Work out the finished part from the listing and answer in its coordinate system (mm). Coordinates: 2 decimals unless noted, no trailing zeros. Order: outer loops, then holes, each group sorted by start corner. A loop starts at its lowest first (then second) coordinate and runs counter-clockwise, first axis right, second up.
```python
from build123d import *

# Parameters (mm, degrees)
CROQUIS1_R              = 6.35
SALIENTE_EXTRUIR1_DEPTH = 12
CROQUIS2_R              = 52.802243625
CROQUIS2_R_2            = 9.5
CORTAR_EXTRUIR1_DEPTH   = 12
CORTAR_EXTRUIR1_DRAFT   = -55
CROQUIS3_R              = 41.337917096
CROQUIS3_R_2            = 9.5
CORTAR_EXTRUIR2_DEPTH   = 12
CORTAR_EXTRUIR2_DRAFT   = -63
CORTAR_EXTRUIR3_REACH   = 20.83
MATRIZC1_COUNT          = 6


with BuildPart() as part:
    # Croquis1 → Saliente-Extruir1 (new body)
    with BuildSketch(Plane(origin=(0, 0, 0), x_dir=(1, 0, 0), z_dir=(0, 1, 0))):
        Polygon((10.969655115, 0), (5.484827557, 9.5), (-5.484827557, 9.5), (-10.969655115, 0), (-5.484827557, -9.5), (5.484827557, -9.5), align=None)
        with Locations(Location((0, 0, 0), (0, 0, 270))):
            Circle(CROQUIS1_R, mode=Mode.SUBTRACT)
    extrude(amount=SALIENTE_EXTRUIR1_DEPTH)


with BuildPart() as cortar_extruir1_tool:
    # Croquis2 → Cortar-Extruir1 (with draft: the straight prism first)
    with BuildSketch(Plane(origin=(0, 12, 0), x_dir=(1, 0, 0), z_dir=(0, 1, 0))):
        Circle(CROQUIS2_R)
        Circle(CROQUIS2_R_2, mode=Mode.SUBTRACT)
    extrude(amount=-CORTAR_EXTRUIR1_DEPTH)
    # Cortar-Extruir1: the draft: its side faces are tilted about the plane it starts from
    cortar_extruir1_sides = [cortar_extruir1_tool.faces().sort_by_distance(p)[0] for p in [
        (-52.802243625, 6, 0),
        (-9.5, 6, 0),
    ]]
    draft(cortar_extruir1_sides, Plane(origin=(0, 12, 0), x_dir=(1, 0, 0), z_dir=(0, 1, 0)), CORTAR_EXTRUIR1_DRAFT)


with BuildPart() as part_1:
    add(part.part)

    # Cortar-Extruir1: cut by cortar_extruir1_tool
    add(cortar_extruir1_tool.part, mode=Mode.SUBTRACT)


with BuildPart() as cortar_extruir2_tool:
    # Croquis3 → Cortar-Extruir2 (with draft: the straight prism first)
    with BuildSketch(Plane.XZ):
        Circle(CROQUIS3_R)
        Circle(CROQUIS3_R_2, mode=Mode.SUBTRACT)
    extrude(amount=-CORTAR_EXTRUIR2_DEPTH)
    # Cortar-Extruir2: the draft: its side faces are tilted about the plane it starts from
    cortar_extruir2_sides = [cortar_extruir2_tool.faces().sort_by_distance(p)[0] for p in [
        (-41.337917096, 6, 0),
        (-9.5, 6, 0),
    ]]
    draft(cortar_extruir2_sides, Plane.XZ, CORTAR_EXTRUIR2_DRAFT)


with BuildPart() as part_2:
    add(part_1.part)

    # Cortar-Extruir2: cut by cortar_extruir2_tool
    add(cortar_extruir2_tool.part, mode=Mode.SUBTRACT)

    # Cortar-Extruir3: up to this cone (the profile starts inside it)
    cortar_extruir3_end = Plane(origin=(0, 12, 0), z_dir=(0, 1, 0)).offset(-16.84049077) * Cone(1.963e-06, 139.780687907, 71.221816836, align=(Align.CENTER, Align.CENTER, Align.MIN), mode=Mode.PRIVATE)
    # Croquis4 → Cortar-Extruir3 (cut, up to the surface)
    with BuildSketch(Plane(origin=(0, 12, 0), x_dir=(1, 0, 0), z_dir=(0, 1, 0)), mode=Mode.PRIVATE) as cortar_extruir3_sk1:
        Polygon((-5.359827557, 9.283493649), (-6.723359894, 8.496257887), (-7.318521333, 9.527107738), (-4.730369323, 11.021377998), (-4.135207884, 9.990528147), align=None)
    cortar_extruir3_tool1 = extrude(cortar_extruir3_sk1.sketch, amount=-CORTAR_EXTRUIR3_REACH, mode=Mode.PRIVATE) & cortar_extruir3_end
    cortar_extruir3 = cortar_extruir3_tool1.solids().sort_by_distance((-5.726865, 12, -9.758818))[0]
    add(cortar_extruir3, mode=Mode.SUBTRACT)

    # MatrizC1: Cortar-Extruir3 ×6 about axis
    matrizc1_axis = Axis((0, 12, 0), (0, 1, 0))
    for i in range(1, MATRIZC1_COUNT):
        add(cortar_extruir3.rotate(matrizc1_axis, i * 360 / MATRIZC1_COUNT), mode=Mode.SUBTRACT)


solid = part_2.part
```
1. Consider probe 1 along X at (y, z) = (10.75, 8); probe 2 along Z at (x, y) = (5, 4.25); probe 3 along Z at (x, y) = (-4, 9.75). Determine where each line is inside the solid, lowest interval first.
2. The mould has two halves that part along Z. Classify faces 1 (the cylindrical face through (-3.86, 5.92, -5.04)), 2 (the flat face through (2, 12, 6.2)), 3 (the conical face through (4.98, 0.17, 8.48)): released by +Z, released by -Z, zero draft, split by the parting line, or undercut.
3. Flat-ended cylindrical pins translate along their axes: pin 1 (5 mm diameter, centred on x = -2.5, z = -1, fed in from +Y); pin 2 (4 mm diameter, centred on x = 7.5, y = 7, fed in from -Z); pin 3 (3 mm diameter, centred on x = 8.5, y = 7.5, fed in from -Z). Find the tip coordinate at first contact, or state that the pin passes through.
4. The part is cut by section A-A (y = 2.75). Determine the outline of the cut face in (x, z), plus the area to 3 significant figures.
Worked out:
1. probe 1: x = -6.35 to 6.35
1. probe 2: z = -9.49 to -3.91, 3.91 to 9.49
1. probe 3: z = -9.5 to -4.93, 4.93 to 9.5
2. face 1: undercut
2. face 2: zero draft
2. face 3: released by +Z
3. pin 1: passes through
3. pin 2: stops at z = -9.2
3. pin 3: stops at z = -6.88
4. outline: (-10.72, -0.43) - (-5.73, -9.07) - (-4.98, -9.5) - (4.98, -9.5) - (5.73, -9.07) - (10.72, -0.43) - (10.72, 0.43) - (5.73, 9.07) - (4.98, 9.5) - (-4.98, 9.5) - (-5.73, 9.07) - (-10.72, 0.43) - close; hole circle Ø12.7 at (0, 0)
4. area: 185 mm2
